Input: dimensioned drawing with shaded views. Units: mm. Origin: part minimum x, y, z. A direction names the side the tool comes from. Round coordinates to 2 decimals unless told otherwise and drop trailing zeros. Loops run counter-clockwise (first coordinate to the right, second up) from the corner with the lowest first, then second, coordinate; pieces in that order, holes last. Notation, with made-up numbers: (-35.5, 11.5) - (3.5, 11.5) arc R15 ccw to (3.5, 40.5) - close; hole circle Ø9 at (89.5, -25.75). An arc over 180 degrees is marked (long way). One line per question, with ' | ' between items. Start each with the question number.
Item 1: Section A-A, the plane y = 12.5. Return loops of the section in (x, z).
Item 2: Section C-C, the plane z = 11. Return loops of the section in (x, y).
Item 3: Section D-D, the plane z = 92. Return loops of the section in (x, y), plus the area to 3 significant figures.
Item 4: Section B-B, the plane x = 12.5. Return loops of the section in (y, z).
Item 5: Material intervals for line 1 along Z through (x, y) = (15.75, 12.5); line 2 along Y through (x, z) = (13, 49); line 3 along Z through (x, y) = (22, 18.75), sorted ascending.
Item 6: Set-up query: the marked faces 1 and 2. Return all of +Z, -Z, +X, -X, +Y, -Y with unobstructed straight access to the full face (end or side cutting, diameter ignored); none if empty.
Item 7: First-contact query: pin 1 (10 mm diameter, centred on y = 2.5, z = 81.5, fed in from +X) (3 decimals); pin 2 (3 mm diameter, centred on y = 6, z = 91.5, fed in from -X) (3 decimals); pin 3 (2 mm diameter, centred on y = 19.5, z = 93, fed in from +X). Flat tips, straight axial feed; report the tip coordinate or a pass-through.
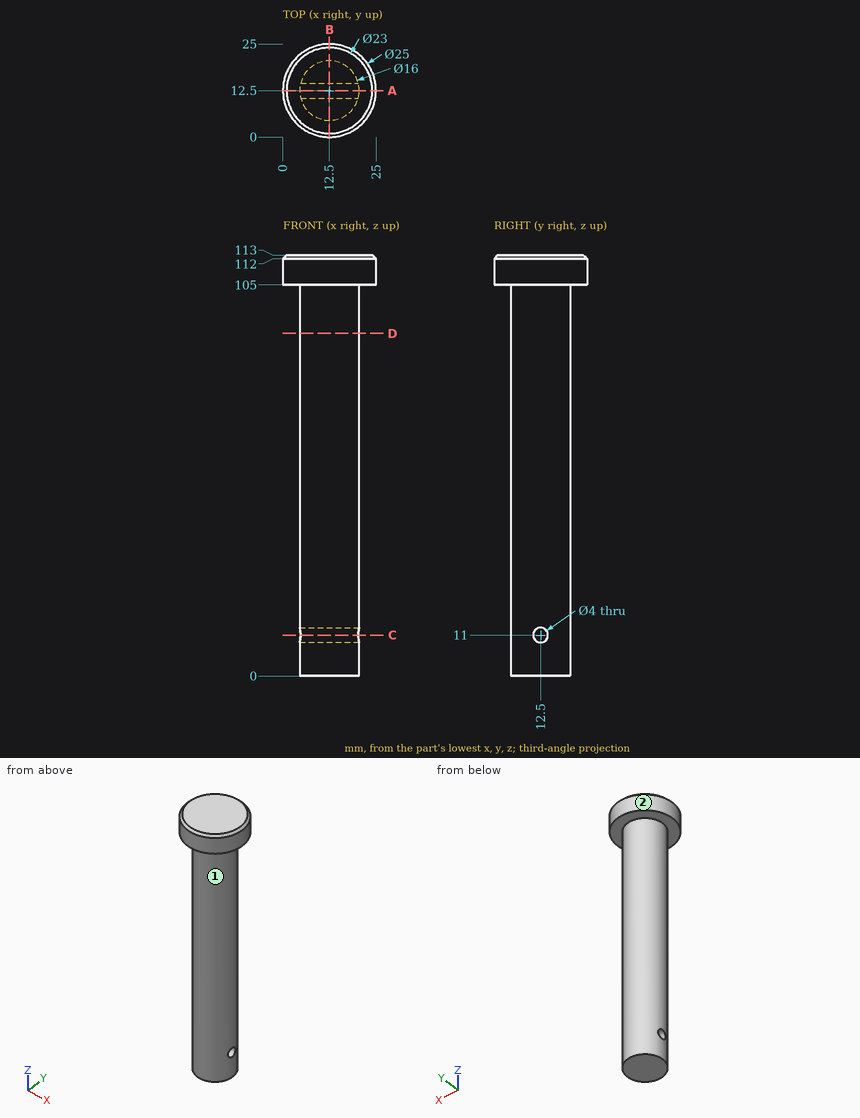
Return value:
1) outline: (0, 105) - (4.5, 105) - (4.5, 13) - (20.5, 13) - (20.5, 105) - (25, 105) - (25, 112) - (24, 113) - (1, 113) - (0, 112) - close; (4.5, 0) - (20.5, 0) - (20.5, 9) - (4.5, 9) - close
2) outline: (4.75, 10.5) arc R8 ccw to (20.25, 10.5) - close; (4.75, 14.5) - (20.25, 14.5) arc R8 ccw to start
3) outline: circle Ø16 at (12.5, 12.5) | area: 201 mm2
4) outline: (0, 105) - (4.5, 105) - (4.5, 0) - (20.5, 0) - (20.5, 105) - (25, 105) - (25, 112) - (24, 113) - (1, 113) - (0, 112) - close; hole circle Ø4 at (12.5, 11)
5) line 1: 0 to 9, 13 to 113 | line 2: 4.52 to 20.48 | line 3: 105 to 113
6) face 1: -Z | face 2: +Z, -Z
7) pin 1: x = 18.745 | pin 2: x = 6.255 | pin 3: x = 17.79
